Autodesk Inventor part; units mm, degrees
ref_plane "YZ Plane" through (0, 0, 0) normal (1, 0, 0) x (0, 1, 0)
ref_plane "XZ Plane" through (0, 0, 0) normal (0, 1, 0) x (-1, 0, 0)
ref_plane "XY Plane" through (0, 0, 0) normal (0, 0, 1) x (1, 0, 0)
sketch "Sketch2" plane through (0, 0, 0) normal (0, 0, 1) x (1, 0, 0)
  circle A0 centre (0, 0) radius 12.7
  circle A1 centre (0, 0) radius 6.35
  line L0 (5.601, 4.732) -> (6.8985, -2.4846)
  line L1 (6.8985, -2.4846) -> (1.2975, -7.2166)
  line L2 (1.2975, -7.2166) -> (-5.601, -4.732)
  line L3 (-5.601, -4.732) -> (-6.8985, 2.4846)
  line L4 (-6.8985, 2.4846) -> (-1.2975, 7.2166)
  line L5 (-1.2975, 7.2166) -> (5.601, 4.732)
  point P0 (2.1518, 5.9743)
  dimension "d8" = 12.7
  dimension "d7" = 25.4
extrude "Extrusion1" add sketch "Sketch2" along normal blind 101.6
properties part number "4-bar intake mid roller"
The model under review builds one solid part; all positions refer to its coordinate system, in mm. A direction names the side the tool comes from. Give positions to 0.01 mm unless a question says otherwise; leave off trailing zeros. Write each loop counter-clockwise with the first axis right and the second up, starting at its lowest first coordinate (ties: lowest second). Pieces come first, ordered by that corner, then holes. Notation, with made-up numbers: M 4,71.5 L 16,71.5 A16 cw 16,87.5 Z; hole C 82,18.5 d9. An arc over 180 degrees is marked long. Write item = value, one per line. Start each with the question number.
Q1. We need section A-A (y = 0). State the section outline as (x, z) points.
Q2. Clearance check with flat-ended pins moving along their axes: pin 1 (10 mm diameter, centred on x = 6, z = 18.5, fed in from -Y); pin 2 (3 mm diameter, centred on x = 3, z = 23.5, fed in from +Y); pin 3 (10 mm diameter, centred on x = -7, z = 42.5, fed in from +Y). State where each tip first meets the part, or that it passes through.
Q3. We need section C-C (z = 37). State the section outline as (x, y) points, plus the area to 3 significant figures.
Q4. Mouldability with a two-part tool opening along X and no side actions: class faces 3 (the face through (3, 6, 0)), 4 (the face through (6.24, 1.17, 50.09)), 5 (the face through (-2.75, 12.4, 50.09)) as released by +X, released by -X, zero draft, split by the parting line, or undercut.
Q5. We need section D-D (y = 8.25). State the section outline as (x, z) points, plus the area to 3 significant figures.
Q6. Machinability: for faces 1 (the face through (3, 6, 101.6)), 2 (the face through (-6.24, -1.17, 50.09)), which of the approach directions +Z, -Z, +X, -X, +Y, -Y give a long, thin tool a straight path to every point of the face, cutting with its end or side? Answer none if there is none.
Q7. We need section B-B (x = 0). State the section outline as (y, z) points.
Q8. For line 1 (X direction, y = -2.75, z = 14.5); line 2 (X direction, y = -3, z = 46); line 3 (Y direction, x = 3.5, z = 90), list the stretches that pass through material, from the lowest coordinate up.
Result set:
q1.outline = M -12.7,0 L -6.45,0 L -6.45,101.6 L -12.7,101.6 Z; M 6.45,0 L 12.7,0 L 12.7,101.6 L 6.45,101.6 Z
q2.pin_1 = -12.66
q2.pin_2 = 12.61
q2.pin_3 = 12.54
q3.outline = C 0,0 d25.4; hole M -6.9,2.48 L -5.6,-4.73 L 1.3,-7.22 L 6.9,-2.48 L 5.6,4.73 L -1.3,7.22 Z
q3.area = 367 mm2
q4.face_3 = zero draft
q4.face_4 = undercut
q4.face_5 = split by the parting line
q5.outline = M -9.66,0 L 9.66,0 L 9.66,101.6 L -9.66,101.6 Z
q5.area = 1,960 mm2
q6.face_1 = +Z, +X, -X, +Y, -Y
q6.face_2 = +Z, -Z
q7.outline = M -12.7,0 L -6.75,0 L -6.75,101.6 L -12.7,101.6 Z; M 6.75,0 L 12.7,0 L 12.7,101.6 L 6.75,101.6 Z
q8.line_1 = -12.4 to -5.96, 6.58 to 12.4
q8.line_2 = -12.34 to -5.91, 6.29 to 12.34
q8.line_3 = -12.21 to -5.36, 5.49 to 12.21
